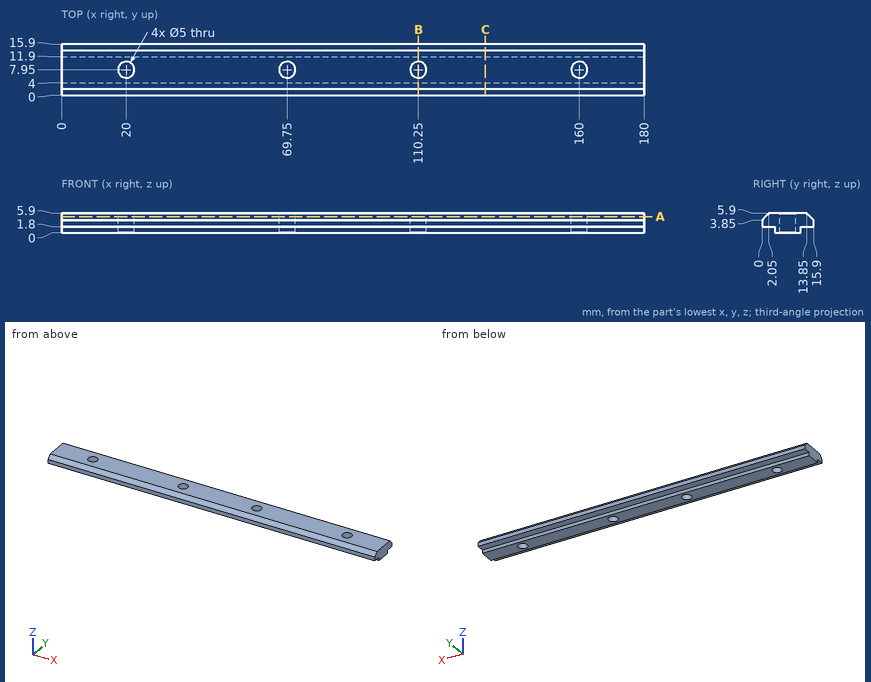
Job drawing, mm, ordinate dimensions from the low corner. One solid piece. Give positions to 0.01 mm unless a question says otherwise; leave off trailing zeros. Loops run counter-clockwise (first coordinate to the right, second up) from the corner with the lowest first, then second, coordinate; pieces in that order, holes last. Notation, with made-up numbers: M 80,-13 L 114,-13 A16 cw 114,5 Z; hole C 66,70 d6. An arc over 180 degrees is marked long. Put each result on its own line as item: value. Start each with the question number.
1) Probe probe 1 along Y at (x, z) = (160, 1.85); probe 2 along X at (y, z) = (6.5, 2.9); probe 3 along Y at (x, z) = (110.25, 1.45). List the from-to ranges inside material, lowest first.
2) Saw through at A-A (z = 4.95). List the corners of the cut face in (x, y).
3) Saw through at C-C (x = 131). List the corners of the cut face in (y, z), then the cut area to 3 significant figures.
4) Saw through at B-B (x = 110.25). List the corners of the cut face in (y, z).
5) Flat gauge pins, fed straight in: pin 1 (1.4 mm diameter, centred on x = 70.5, z = 1, fed in from +Y); pin 2 (2 mm diameter, centred on x = 122.5, y = 1.5, fed in from -Z); pin 3 (4 mm diameter, centred on x = 110.25, y = 7.95, fed in from +Z) (3 decimals); pin 4 (1.4 mm diameter, centred on x = 110, z = 1, fed in from -Y). Where does each tip first touch, or does it go through?
Numbers:
1. probe 1: 0 to 5.45, 10.45 to 15.9
1. probe 2: 0 to 17.96, 22.04 to 67.71, 71.79 to 108.21, 112.29 to 157.96, 162.04 to 180
1. probe 3: 4 to 5.45, 10.45 to 11.9
2. outline: M 0,1.1 L 180,1.1 L 180,14.8 L 0,14.8 Z; hole C 20,7.95 d5; hole C 69.75,7.95 d5; hole C 110.25,7.95 d5; hole C 160,7.95 d5
3. outline: M 0,1.8 L 4,1.8 L 4,0 L 11.9,0 L 11.9,1.8 L 15.9,1.8 L 15.9,3.85 L 13.85,5.9 L 2.05,5.9 L 0,3.85 Z
3. area: 75.2 mm^2
4. outline: M 0,1.8 L 4,1.8 L 4,0 L 5.45,0 L 5.45,5.9 L 2.05,5.9 L 0,3.85 Z; M 10.45,0 L 11.9,0 L 11.9,1.8 L 15.9,1.8 L 15.9,3.85 L 13.85,5.9 L 10.45,5.9 Z
5. pin 1: y = 11.9
5. pin 2: z = 1.8
5. pin 3: through
5. pin 4: y = 4
